Autodesk Inventor part; units mm, degrees
ref_plane "YZ Plane" through (0, 0, 0) normal (1, 0, 0) x (0, 1, 0)
ref_plane "XZ Plane" through (0, 0, 0) normal (0, 1, 0) x (-1, 0, 0)
ref_plane "XY Plane" through (0, 0, 0) normal (0, 0, 1) x (1, 0, 0)
sketch "草圖2" plane through (0, 0, 0) normal (0, 1, 0) x (-1, 0, 0)
  line L0 (-2.8868, 0) -> (-1.4434, 2.5)
  line L1 (-1.4434, 2.5) -> (1.4434, 2.5)
  line L2 (1.4434, 2.5) -> (2.8868, 0)
  line L3 (2.8868, 0) -> (1.4434, -2.5)
  line L4 (1.4434, -2.5) -> (-1.4434, -2.5)
  line L5 (-1.4434, -2.5) -> (-2.8868, 0)
  point P0 (0, 0)
  point P1 (0, 0)
  dimension "d2" = 5
extrude "擠出1" add sketch "草圖2" along normal blind 4
sketch "草圖3" plane through (0, 0, 0) normal (0, 0, 1) x (1, 0, 0)
  line L0 (1.4434, 4) -> (-1.4434, 4)
  line L1 (0, 4) -> (1.5, 4)
  line L2 (1.5, 4) -> (1.5, 10)
  line L3 (1.5, 10) -> (0, 10)
  line L4 (0, 10) -> (0, 4)
  line L5 (0, 17.268) -> (0, -3.3114)
  line L6 (0, 0) -> (1.5, 0)
  line L7 (1.5, 0) -> (1.5, -6)
  line L8 (1.5, -6) -> (0, -6)
  line L9 (0, -6) -> (0, 0)
  point P0 (0.75, 10)
  dimension "d5" = 3
  dimension "d6" = 6
  dimension "d8" = 6
revolve "迴轉1" add sketch "草圖3" angle 360 about axis through (0, 17.268, 0) along (0, -1, 0)
properties part number "copper_pillar_M3_L15" material "Copper"
Source: CAD feature listing. Evaluate the final solid. Frame: model axes, mm. A direction names the side the tool comes from. Round coordinates to 2 decimals unless told otherwise and drop trailing zeros. Write each loop counter-clockwise with the first axis right and the second up, starting at its lowest first coordinate (ties: lowest second). Pieces come first, ordered by that corner, then holes. Notation, with made-up numbers: (47, -4.5) - (89, -4.5) arc R22 cw to (89, 24.5) - close; hole circle Ø2 at (-3, 45.5). An arc over 180 degrees is marked (long way). Use CSV: the item, a comma, the result in double quotes. Start each with the question number.
(1) Cut plane C-C, the plane y = -2.25. Return loops of the section in (x, z), and give its area (3 significant figures).
(2) Cut plane A-A, the plane x = 0. Return loops of the section in (y, z).
(3) Cut plane D-D, the plane x = -1.7. Return loops of the section in (y, z).
(4) First-contact query: pin 1 Ø1.5 at (x, z) = (0.5, 1.5) entering from -Y; pin 2 Ø2 at (x, y) = (1.5, 7) entering from +Z; pin 3 Ø1 at (y, z) = (8.5, 0.5) entering from -X. Flat tips, straight axial feed; report the tip coordinate or a pass-through.
(5) Set-up query: faces 1 (the face through (-1.5, -3.04, 0.07)), 2 (the face through (0, 10, 0)), 3 (the face through (-1.24, 4, 1.15)). Return all of +Z, -Z, +X, -X, +Y, -Y with unobstructed straight access to the full face (end or side cutting, diameter ignored); none if empty.
(6) Cut plane B-B, the plane z = -1.3. Return loops of the section in (x, y).
(7) Material intervals for probe 1 along Y at (x, z) = (-2.5, -0.6); probe 2 along X at (y, z) = (1.5, -2.15); probe 3 along X at (y, z) = (-3.5, 0.5), sorted ascending. Write a range as [from, to].
Geometry says:
1,outline,"circle Ø3 at (0, 0)"
1,area,"7.07 mm²"
2,outline,"(-6, -1.5) - (0, -1.5) - (0, -2.5) - (4, -2.5) - (4, -1.5) - (10, -1.5) - (10, 1.5) - (4, 1.5) - (4, 2.5) - (0, 2.5) - (0, 1.5) - (-6, 1.5) - close"
3,outline,"(0, -2.06) - (4, -2.06) - (4, 2.06) - (0, 2.06) - close"
4,pin 1,"y = -6"
4,pin 2,"z = 1.41"
4,pin 3,"x = -1.5"
5,face 1,"-Y"
5,face 2,"+Z, -Z, +X, -X, +Y"
5,face 3,"+Y"
6,outline,"(-2.14, 0) - (-0.75, 0) - (-0.75, -6) - (0.75, -6) - (0.75, 0) - (2.14, 0) - (2.14, 4) - (0.75, 4) - (0.75, 10) - (-0.75, 10) - (-0.75, 4) - (-2.14, 4) - close"
7,probe 1,"[0, 4]"
7,probe 2,"[-1.65, 1.65]"
7,probe 3,"[-1.41, 1.41]"
